The model under review builds one solid part; all positions refer to its coordinate system, in mm. A direction names the side the tool comes from. Round coordinates to 2 decimals unless told otherwise and drop trailing zeros. Order: outer loops, then holes, each group sorted by start corner. A loop starts at its lowest first (then second) coordinate and runs counter-clockwise, first axis right, second up. Notation, with made-up numbers: M 69.25,62 L 114.25,62 A17 cw 114.25,74 Z; hole C 29.5,39.5 d2. An arc over 180 degrees is marked long. Answer as a JSON object with one key per item and string values. Group by question number.
1. To check wall thickness, follow probe 1 along X at (y, z) = (19, 30); probe 2 along X at (y, z) = (0.5, 6.5); probe 3 along Z at (x, y) = (21, 7). State the ranges of each line that lie inside material, in increasing order. Write a range as [from, to].
2. Add section A-A on y = 19. State the section outline as (x, z) points.
3. Add section C-C on x = 28. State the section outline as (y, z) points.
4. Add section B-B on z = 21.5. State the section outline as (x, y) points.
5. Machinability: for faces 4 (the face through (43.706, -6, 17)), 5 (the face through (43, 10.268, 17)), 6 (the face through (-31, 33.126, 17)), which of the approach directions +Z, -Z, +X, -X, +Y, -Y give a long, thin tool a straight path to every point of the face, cutting with its end or side? Answer none if there is none.
6. Mouldability with a two-part tool opening along X and no side actions: class faces 1 (the face through (51.206, 19, 17)), 2 (the face through (-28.794, 21, 17)), 3 (the face through (-30, 5.126, 17)) as released by +X, released by -X, zero draft, split by the parting line, or undercut.
7. Clearance check with flat-ended pins moving along their axes: P1, Ø4, axis at x = 19.5, y = 5.5, coming from the -Z side; P2, Ø6.5, axis at y = -4, z = 20.5, coming from the -X side; P3, Ø5.5, axis at x = -30.5, z = 11.5, coming from the +Y side. State where each tip first meets the part, or that it passes through.
8. Add section D-D on z = 13. State the section outline as (x, y) points, and give its area (3 significant figures).
```python
from build123d import *

# Parameters (mm, degrees)
EXTRUDE_1_DEPTH     = 35
EXTRUDE_2_DEPTH     = 3
SKETCH_3_R          = 1.45
CUT_EXTRUDE_1_DEPTH = 98.758571233


with BuildPart() as part:
    # 草圖1 → 填料-伸長1 (new body)
    with BuildSketch(Plane.XY):
        Polygon((-21.293611747, 10.125539125), (-28.793611747, 10.125539125), (-28.793611747, 33.125539125), (-33.793611747, 33.125539125), (-33.793611747, 5.125539125), (-26.293611747, 5.125539125), (-26.293611747, -16.732324255), (43.706388253, -16.732324255), (43.706388253, 5.267675745), (51.206388253, 5.267675745), (51.206388253, 33.267675745), (46.206388253, 33.267675745), (46.206388253, 10.267675745), (38.706388253, 10.267675745), (38.706388253, -11.732324255), (-21.293611747, -11.732324255), align=None)
    extrude(amount=EXTRUDE_1_DEPTH)

    # 草圖2 → 填料-伸長2 (add)
    with BuildSketch(Plane.XY.offset(35)):
        Polygon((51.206388253, 10.125539125), (51.206388253, 5.267675745), (43.706388253, 5.267675745), (43.706388253, -16.732324255), (-26.293611747, -16.732324255), (-26.293611747, 5.125539125), (-33.793611747, 5.125539125), (-33.793611747, 10.125539125), align=None)
    extrude(amount=-EXTRUDE_2_DEPTH)

    # 草圖3 → 除料-伸長1 (cut, through all)
    with BuildSketch(Plane.ZY.offset(33.793611747)):
        with Locations(Location((6.5, 28.407675745, 0), (0, 0, 270))):
            Circle(SKETCH_3_R)
        with Locations(Location((21.5, 28.407675745, 0), (0, 0, 270))):
            Circle(SKETCH_3_R)
    extrude(amount=-CUT_EXTRUDE_1_DEPTH, mode=Mode.SUBTRACT)


solid = part.part
```
Recorded:
{
 "1": {"probe 1": "x = [-33.79, -28.79], [46.21, 51.21]", "probe 2": "x = [-26.29, -21.29], [38.71, 43.71]", "probe 3": "z = [32, 35]"},
 "2": {"outline": "M -33.79,0 L -28.79,0 L -28.79,35 L -33.79,35 Z; M 46.21,0 L 51.21,0 L 51.21,35 L 46.21,35 Z"},
 "3": {"outline": "M -16.73,0 L -11.73,0 L -11.73,32 L 10.13,32 L 10.13,35 L -16.73,35 Z"},
 "4": {"outline": "M -33.79,5.13 L -26.29,5.13 L -26.29,-16.73 L 43.71,-16.73 L 43.71,5.27 L 51.21,5.27 L 51.21,26.96 L 46.21,26.96 L 46.21,10.27 L 38.71,10.27 L 38.71,-11.73 L -21.29,-11.73 L -21.29,10.13 L -28.79,10.13 L -28.79,26.96 L -33.79,26.96 Z; M -33.79,29.86 L -28.79,29.86 L -28.79,33.13 L -33.79,33.13 Z; M 46.21,29.86 L 51.21,29.86 L 51.21,33.27 L 46.21,33.27 Z"},
 "5": {"face 4": "+Z, -Z, +X, -Y", "face 5": "+Z, -Z, +Y", "face 6": "+Z, -Z, -X, +Y"},
 "6": {"face 1": "released by +X", "face 2": "undercut", "face 3": "zero draft"},
 "7": {"P1": "stops at z = 32", "P2": "stops at x = -26.29", "P3": "stops at y = 33.13"},
 "8": {"outline": "M -33.79,5.13 L -26.29,5.13 L -26.29,-16.73 L 43.71,-16.73 L 43.71,5.27 L 51.21,5.27 L 51.21,33.27 L 46.21,33.27 L 46.21,10.27 L 38.71,10.27 L 38.71,-11.73 L -21.29,-11.73 L -21.29,10.13 L -28.79,10.13 L -28.79,33.13 L -33.79,33.13 Z", "area": "874 mm²"}
}
